from build123d import *

# Parameters (mm, degrees)
MODEL_W         = 13.9993
MODEL_H         = 13.99946
MODEL_W_2       = 13.99955
MODEL_H_2       = 13.9994
MODEL_H_3       = 13.9993
EXTRUDE_1_DEPTH = 2


with BuildPart() as part:
    # Model → 凸台-拉伸1 (new body)
    with BuildSketch(Plane.XY):
        Polygon((-0.38035, 95.9831), (76.769, 95.9831), (76.769, 80.38337), (79.769, 80.38337), (79.769, 75.38337), (76.769, 75.38337), (76.769, 50.38337), (79.769, 50.38337), (79.769, 45.38337), (76.769, 45.38337), (76.769, 20.38337), (79.769, 20.38337), (79.769, 15.38337), (76.769, 15.38337), (76.769, -0.21636), (-0.38035, -0.21636), (-0.38035, 15.38337), (-3.38035, 15.38337), (-3.38035, 20.38337), (-0.38035, 20.38337), (-0.38035, 45.38337), (-3.38035, 45.38337), (-3.38035, 50.38337), (-0.38035, 50.38337), (-0.38035, 75.38337), (-3.38035, 75.38337), (-3.38035, 80.38337), (-0.38035, 80.38337), align=None)
        Polygon((12.1447, 16.7831), (12.1447, 12.0826), (10.6192, 12.0826), (10.6192, 15.3128), (3.86955, 15.3128), (3.86955, 12.0826), (3.04409, 12.0826), (3.04409, 9.28384), (3.86955, 9.28384), (3.86955, 3.01377), (5.59484, 3.01377), (5.59484, 1.8135), (8.89385, 1.8135), (8.89385, 3.01377), (10.6192, 3.01377), (10.6192, 7.48273), (12.1447, 7.48273), (12.1447, 2.78364), (26.1441, 2.78364), (26.1441, 7.48273), (27.6696, 7.48273), (27.6696, 3.01377), (29.3949, 3.01377), (29.3949, 1.8135), (32.694, 1.8135), (32.694, 3.01377), (34.4193, 3.01377), (34.4193, 9.28384), (35.2447, 9.28384), (35.2447, 12.0826), (34.4193, 12.0826), (34.4193, 15.3128), (27.6696, 15.3128), (27.6696, 12.0826), (26.1441, 12.0826), (26.1441, 16.7831), align=None, mode=Mode.SUBTRACT)
        with Locations((47.71935, 9.78337)):
            Rectangle(MODEL_W, MODEL_H, mode=Mode.SUBTRACT)
        Polygon((66.27, 35.4087), (66.27, 34.5833), (59.9997, 34.5833), (59.9997, 32.8579), (58.7996, 32.8579), (58.7996, 29.5589), (59.9997, 29.5589), (59.9997, 27.8336), (64.4701, 27.8336), (64.4701, 26.3081), (59.7697, 26.3081), (59.7697, 12.3086), (64.4701, 12.3086), (64.4701, 10.7831), (59.9997, 10.7831), (59.9997, 9.05785), (58.7996, 9.05785), (58.7996, 5.75881), (59.9997, 5.75881), (59.9997, 4.03352), (66.27, 4.03352), (66.27, 3.20807), (69.07, 3.20807), (69.07, 4.03352), (72.3, 4.03352), (72.3, 10.7831), (69.07, 10.7831), (69.07, 12.3086), (73.769, 12.3086), (73.769, 26.3081), (69.07, 26.3081), (69.07, 27.8336), (72.3, 27.8336), (72.3, 34.5833), (69.07, 34.5833), (69.07, 35.4087), align=None, mode=Mode.SUBTRACT)
        with Locations((9.619425, 28.8333)):
            Rectangle(MODEL_W_2, MODEL_H_2, mode=Mode.SUBTRACT)
        with Locations((28.66935, 28.8333)):
            Rectangle(MODEL_W, MODEL_H_2, mode=Mode.SUBTRACT)
        with Locations((47.71935, 28.8333)):
            Rectangle(MODEL_W, MODEL_H_2, mode=Mode.SUBTRACT)
        with Locations((9.619425, 47.88345)):
            Rectangle(MODEL_W_2, MODEL_H_3, mode=Mode.SUBTRACT)
        with Locations((28.66935, 47.88345)):
            Rectangle(MODEL_W, MODEL_H_3, mode=Mode.SUBTRACT)
        with Locations((47.71935, 47.88345)):
            Rectangle(MODEL_W, MODEL_H_3, mode=Mode.SUBTRACT)
        Polygon((66.27, 73.5087), (66.27, 72.6832), (59.9997, 72.6832), (59.9997, 70.9581), (58.7996, 70.9581), (58.7996, 67.6589), (59.9997, 67.6589), (59.9997, 65.9335), (64.4701, 65.9335), (64.4701, 64.4081), (59.7697, 64.4081), (59.7697, 50.4088), (64.4701, 50.4088), (64.4701, 48.883), (59.9997, 48.883), (59.9997, 47.1579), (58.7996, 47.1579), (58.7996, 43.8587), (59.9997, 43.8587), (59.9997, 42.1337), (66.27, 42.1337), (66.27, 41.3082), (69.07, 41.3082), (69.07, 42.1337), (72.3, 42.1337), (72.3, 48.883), (69.07, 48.883), (69.07, 50.4088), (73.769, 50.4088), (73.769, 64.4081), (69.07, 64.4081), (69.07, 65.9335), (72.3, 65.9335), (72.3, 72.6832), (69.07, 72.6832), (69.07, 73.5087), align=None, mode=Mode.SUBTRACT)
        with Locations((9.619425, 66.93345)):
            Rectangle(MODEL_W_2, MODEL_H_3, mode=Mode.SUBTRACT)
        with Locations((28.66935, 66.93345)):
            Rectangle(MODEL_W, MODEL_H_3, mode=Mode.SUBTRACT)
        with Locations((47.71935, 66.93345)):
            Rectangle(MODEL_W, MODEL_H_3, mode=Mode.SUBTRACT)
        with Locations((9.619425, 85.98345)):
            Rectangle(MODEL_W_2, MODEL_H_3, mode=Mode.SUBTRACT)
        with Locations((28.66935, 85.98345)):
            Rectangle(MODEL_W, MODEL_H_3, mode=Mode.SUBTRACT)
        with Locations((47.71935, 85.98345)):
            Rectangle(MODEL_W, MODEL_H_3, mode=Mode.SUBTRACT)
        with Locations((66.76935, 85.98345)):
            Rectangle(MODEL_W, MODEL_H_3, mode=Mode.SUBTRACT)
    extrude(amount=EXTRUDE_1_DEPTH)


solid = part.part
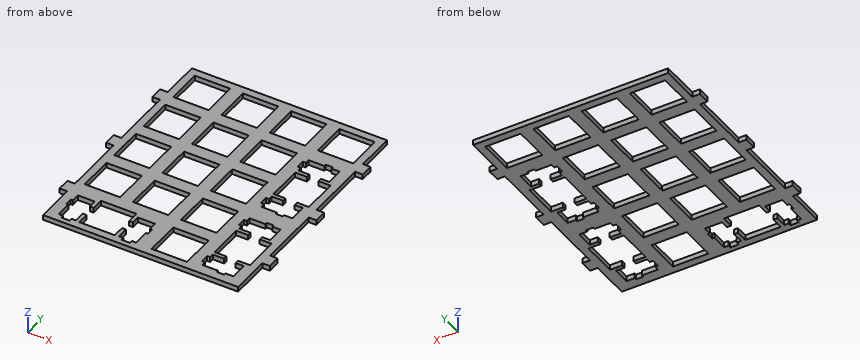
Work out the finished part from the listing and answer in its coordinate system (mm). Round coordinates to 2 decimals unless told otherwise and drop trailing zeros. Write each loop counter-clockwise with the first axis right and the second up, starting at its lowest first coordinate (ties: lowest second). Pieces come first, ordered by that corner, then holes. Notation, with made-up numbers: (35, 77.5) -> (84, 77.5) arc R7 ccw to (84, 87.5) -> close; hole circle Ø1 at (37.25, 9.5). An arc over 180 degrees is marked (long way). Write each question's results on one line, items separated by ' | '.
Item 1: A cutting plane is placed at B-B, the plane x = 43. Determine the outline of the cut face in (y, z).
Result set:
outline: (-0.22, 0) -> (2.78, 0) -> (2.78, 2) -> (-0.22, 2) -> close; (16.78, 0) -> (21.83, 0) -> (21.83, 2) -> (16.78, 2) -> close; (35.83, 0) -> (40.88, 0) -> (40.88, 2) -> (35.83, 2) -> close; (54.88, 0) -> (59.93, 0) -> (59.93, 2) -> (54.88, 2) -> close; (73.93, 0) -> (78.98, 0) -> (78.98, 2) -> (73.93, 2) -> close; (92.98, 0) -> (95.98, 0) -> (95.98, 2) -> (92.98, 2) -> close
Item 2: A cutting plane is placed at A-A, the plane y = 84.5. Determine the outline of the cut face in (x, z).
Result set:
outline: (-0.38, 0) -> (2.62, 0) -> (2.62, 2) -> (-0.38, 2) -> close; (16.62, 0) -> (21.67, 0) -> (21.67, 2) -> (16.62, 2) -> close; (35.67, 0) -> (40.72, 0) -> (40.72, 2) -> (35.67, 2) -> close; (54.72, 0) -> (59.77, 0) -> (59.77, 2) -> (54.72, 2) -> close; (73.77, 0) -> (76.77, 0) -> (76.77, 2) -> (73.77, 2) -> close
Item 3: A cutting plane is placed at C-C, the plane z = 0.55. Count the separate pieces of the cut face and the enclosed holes in it, plus the area to 3 significant figures.
Result set:
separate pieces: 1 | enclosed holes: 17 | area: 3,600 mm^2
Item 4: Flat-ended cylindrical pins translate along their axes: P1, Ø1, axis at y = 9.5, z = 1, coming from the +X side; P2, Ø1, axis at y = 6.5, z = 1, coming from the -X side. Find the tip coordinate at first contact, or state that the pin passes through.
Result set:
P1: x = 76.77 | P2: x = -0.38
Item 5: Find the intervals of material crossed by line 1 along Y through (x, z) = (52.5, 1.5); line 2 along X through (y, z) = (29, 1.15); line 3 along Y through (x, z) = (27.5, 0.85), in increasing order. Write a range as [from, to].
Result set:
line 1: [-0.22, 2.78], [16.78, 21.83], [35.83, 40.88], [54.88, 59.93], [73.93, 78.98], [92.98, 95.98] | line 2: [-0.38, 2.62], [16.62, 21.67], [35.67, 40.72], [54.72, 60], [72.3, 76.77] | line 3: [-0.22, 7.48], [12.08, 21.83], [35.83, 40.88], [54.88, 59.93], [73.93, 78.98], [92.98, 95.98]
